Geometry check sheet. Reference: the model listing, model coordinates, mm. Give positions to 0.01 mm unless a question says otherwise; leave off trailing zeros. Write each loop counter-clockwise with the first axis right and the second up, starting at its lowest first coordinate (ties: lowest second). Pieces come first, ordered by that corner, then holes. Notation, with made-up numbers: (-34.5, 27) -> (-9.5, 27) arc R16 ccw to (-9.5, 36) -> close; hole circle Ø11 at (6.5, 17). An arc over 180 degrees is marked (long way). Write item = value, one per line. Start each with the question number.
1. Depth check by flat-ended pin: P1, Ø1, axis at y = 6, z = 0.5, coming from the +X side. Enter the tip coordinate at first touch or a pass-through.
2. Mould release check, pull along Y, two halves, no side actions. Record for faces 1 (the flat face through (0, 3, 0)), 2 (the cylindrical face through (1.09, 1.94, -0.14)): pulls with the +Y half, pulls with the -Y half, needs draft (parallel to the pull), parting line crosses it, or undercut.
3. Thickness scan on line 1 along Y through (x, z) = (-0.05, 0.1); line 2 along X through (y, z) = (1.25, 0.1); line 3 along Z through (x, y) = (-0.05, 7.25). Record the ranges inside material, lowest first.
4. Cross-section at B-B, the plane y = 2.75. Record the cut outline in (x, z), plus the area to 3 significant figures.
5. Cross-section at A-A, the plane y = 3.75. Record the cut outline in (x, z).
```python
from build123d import *

# Parameters (mm, degrees)
SKETCH_1_R      = 1.1
EXTRUDE_1_DEPTH = 3
FILLET_1_R      = 0.9
SKETCH_2_R      = 0.25
EXTRUDE_2_DEPTH = 5


with BuildPart() as part:
    # 草图1 → 拉伸1 (new body)
    with BuildSketch(Plane(origin=(0, 0, 0), x_dir=(1, 0, 0), z_dir=(0, 1, 0))):
        with Locations(Location((0, 0, 0), (0, 0, 270))):
            Circle(SKETCH_1_R)
    extrude(amount=EXTRUDE_1_DEPTH)

    # 圆角1
    fillet_1_edges = [part.edges().sort_by_distance(p)[0] for p in [
        (0, 0, -1.1),
    ]]
    fillet(fillet_1_edges, radius=FILLET_1_R)

    # 草图2 → 拉伸2 (add)
    with BuildSketch(Plane(origin=(0, 3, 0), x_dir=(-1, 0, 0), z_dir=(0, 1, 0))):
        with Locations(Location((0, -0.5, 0), (0, 0, 90))):
            Circle(SKETCH_2_R)
        with Locations(Location((0, 0.5, 0), (0, 0, 270))):
            Circle(SKETCH_2_R)
    extrude(amount=EXTRUDE_2_DEPTH)


solid = part.part
```
Answers:
q1.P1 = 0.25
q2.face_1 = pulls with the +Y half
q2.face_2 = needs draft
q3.line_1 = 0 to 3
q3.line_2 = -1.1 to 1.1
q3.line_3 = -0.74 to -0.26, 0.26 to 0.74
q4.outline = circle Ø2.2 at (0, 0)
q4.area = 3.80 mm^2
q5.outline = circle Ø0.5 at (0, -0.5); circle Ø0.5 at (0, 0.5)
